Autodesk Fusion 360 part; units mm, degrees
sketch "Sketch1" plane through (0, 0, 0) normal (0, 1, 0) x (1, 0, 0)
  line L0 (20, 0) -> (20, -127)
  line L1 (0, -127) -> (0, 0)
  arc A0 (0, -127) -> (20, -127) centre (10, -127) ccw
  line L2 (0, 0) -> (20, 0)
  circle A1 centre (10, -127) radius 1.6
  dimension "d1" = 20
  dimension "d2" = 127
  dimension "d3" = 3.2
extrude "Extrude1" add sketch "Sketch1" along normal blind 20
sketch "Sketch2" plane through (0, 0, 0) normal (0, 0, -1) x (-1, 0, 0)
  line L0 (-20, 0) -> (0, 0)
  line L1 (0, 0) -> (0, 20)
  line L2 (0, 20) -> (-20, 20)
  line L3 (-20, 20) -> (-20, 0)
  line L4 (-20, 20) -> (0, 20)
  line L5 (0, 20) -> (0, 0)
  line L6 (0, 0) -> (-20, 0)
  line L7 (-20, 0) -> (-20, 20)
  circle A0 centre (-16, 16) radius 1
  circle A1 centre (-4, 16) radius 1
  circle A2 centre (-16, 4) radius 1
  circle A3 centre (-4, 4) radius 1
  dimension "d6" = 2
  dimension "d7" = 2
  dimension "d8" = 2
  dimension "d9" = 2
  dimension "d16" = 4
  dimension "d17" = 4
  dimension "d18" = 4
  dimension "d19" = 4
  dimension "d20" = 4
  dimension "d21" = 4
  dimension "d22" = 4
  dimension "d23" = 4
extrude "Extrude2" cut sketch "Sketch2" against normal blind 40 contours A0 | A1 | A2 | A3
sketch "Sketch3" plane through (0, 20, 0) normal (0, 1, 0) x (-1, 0, 0)
  circle A0 centre (-10, 127) radius 1.6
  arc A1 (0, 127) -> (-20, 127) centre (-10, 127) ccw
  line L0 (-20, 127) -> (-20, 0)
  line L1 (-20, 0) -> (0, 0)
  line L2 (0, 0) -> (0, 127)
  circle A2 centre (-10, 114.3) radius 1.6
  circle A3 centre (-10, 101.6) radius 1.6
  circle A4 centre (-10, 88.9) radius 1.6
  circle A5 centre (-10, 76.2) radius 1.6
  circle A6 centre (-10, 63.5) radius 1.6
  circle A7 centre (-10, 50.8) radius 1.6
  circle A8 centre (-10, 38.1) radius 1.6
  dimension "d24" = 3.2
  dimension "d25" = 12.7
  dimension "d28" = 0
  dimension "d29" = -12.7
extrude "Extrude3" cut sketch "Sketch3" against normal blind 170 contours A2 | A3 | A4 | A5 | A6 | A7 | A8
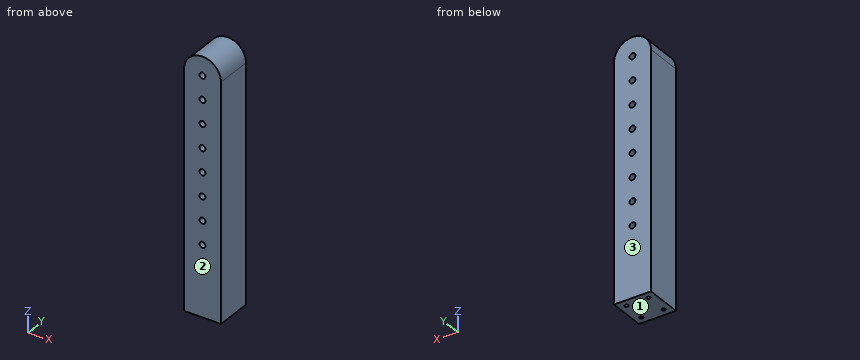
Verification items for the finished model (mm, model axes). Face numbers are marked on the shaded views. Round coordinates to 2 decimals unless told otherwise and drop trailing zeros. Write each loop counter-clockwise with the first axis right and the second up, starting at its lowest first coordinate (ties: lowest second). Pieces come first, ordered by that corner, then holes.
1. Draft check along Y on the marked faces 1, 2 and 3. Enter one of: +Y half, -Y half, draft (parallel to the pull), parting line (faces both ways), or undercut.
2. Gauge pin test, flat ends, axial feed: P1, Ø3, axis at x = 16, y = 16, coming from the +Z side; P2, Ø0.6, axis at x = 3.5, y = 16, coming from the -Z side; P3, Ø2.5, axis at x = 16, y = 4, coming from the +Z side. Record the tip position at first contact, or that the pin passes through.
3. Section check A-A on z = 19.5. Enter the section's corners in (x, y), plus the area to 3 significant figures.
4. Section check B-B on z = 63.5. Enter the section's corners in (x, y), plus the area to 3 significant figures.
5. Scan lines: L1, parallel to Y at x = 16, z = 27; L2, parallel to Y at x = 15.5, z = 30.5; L3, parallel to X at y = 11.5, z = 38. Record each from-to range of solid material in increasing order.
6. Section check C-C on y = 1.5. State how many separate pieces and enclosed holes the cut face has, plus the area to 3 significant figures.
Answer:
1. face 1: draft
1. face 2: -Y half
1. face 3: +Y half
2. P1: stops at z = 135.93
2. P2: stops at z = 40
2. P3: stops at z = 135.8
3. outline: (0, 0) - (20, 0) - (20, 20) - (0, 20) - close; hole circle Ø2 at (4, 4); hole circle Ø2 at (4, 16); hole circle Ø2 at (16, 4); hole circle Ø2 at (16, 16)
3. area: 387 mm2
4. outline: (0, 0) - (8.4, 0) - (8.4, 20) - (0, 20) - close; (11.6, 0) - (20, 0) - (20, 20) - (11.6, 20) - close
4. area: 336 mm2
5. L1: y = 0 to 3, 5 to 15, 17 to 20
5. L2: y = 0 to 3.13, 4.87 to 15.13, 16.87 to 20
5. L3: x = 0 to 8.4, 11.6 to 20
6. separate pieces: 1
6. enclosed holes: 8
6. area: 2,630 mm2
